The listing builds one solid part. Answer for the finished solid, in the listing's coordinates (mm). Face numbers are marked on the shaded views. Round coordinates to 2 decimals unless told otherwise and drop trailing zeros. Order: outer loops, then holes, each group sorted by start corner. A loop starts at its lowest first (then second) coordinate and runs counter-clockwise, first axis right, second up. Notation, with made-up numbers: (67.5, 25) - (73.5, 25) arc R22 ccw to (73.5, 33) - close; hole circle Ø10 at (-13.5, 40.25). An arc over 180 degrees is marked (long way). One line per item, written item: value. Start each with the question number.
1. Section B-B, the plane x = -24 is taken. Give the vertices of the cut face in (y, z).
2. Section A-A, the plane z = 24.5 is taken. Give the vertices of the cut face in (x, y).
3. Straight lines are drawn through the part: line 1 (Z direction, x = 27, y = -2.75); line 2 (Z direction, x = -12.5, y = -18.25); line 3 (Z direction, x = -11, y = -7.5). For each, find the intervals that lie inside material, in ascending order.
4. Section C-C, the plane y = -19.25 is taken. Count the separate pieces of the cut face and the enclosed holes in it, then the cut area to 3 significant figures.
5. For a pull along Z with two mould halves and no side action, classify the marked faces 1, 2, 3 and 4 as released by +Z, released by -Z, zero draft, split by the parting line, or undercut.
6. Section D-D, the plane x = 42.5 is taken. Give the vertices of the cut face in (y, z).
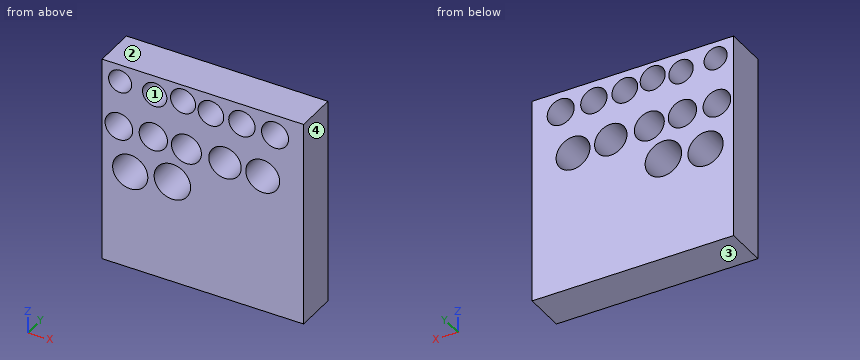
from build123d import *

# Parameters (mm, degrees)
F0_W     = 123.113498
F0_H     = 126.693976
F1_DEPTH = 25.4
F3_D     = 14.1
F4_D     = 14.9
F5_D     = 15.3
F6_D     = 15.7
F7_D     = 16.1
F8_D     = 16.5
F9_D     = 16.9
F10_D    = 17.3
F11_D    = 18.3
F12_D    = 19.8
F13_D    = 20.7
F14_D    = 21.5
F15_D    = 22.3


with BuildPart() as f1:
    # F0 (on Front) → F1 (new body)
    with BuildSketch(Plane.XZ):
        with Locations((2.891928, -3.167348)):
            Rectangle(F0_W, F0_H)
    extrude(amount=F1_DEPTH)

    # F3 (through all)
    with Locations(Plane.XZ.offset(25.4)):
        with Locations((-47.647953, 49.713619)):
            Hole(F3_D / 2)

    # F4 (through all)
    with Locations(Plane.XZ.offset(25.4)):
        with Locations((-26.540603, 48.396926)):
            Hole(F4_D / 2)

    # F5 (through all)
    with Locations(Plane.XZ.offset(25.4)):
        with Locations((-9.222592, 50.100338)):
            Hole(F5_D / 2)

    # F6 (through all)
    with Locations(Plane.XZ.offset(25.4)):
        with Locations((7.811517, 48.113026)):
            Hole(F6_D / 2)

    # F7 (through all)
    with Locations(Plane.XZ.offset(25.4)):
        with Locations((26.720595, 47.939809)):
            Hole(F7_D / 2)

    # F8 (through all)
    with Locations(Plane.XZ.offset(25.4)):
        with Locations((46.989974, 47.545221)):
            Hole(F8_D / 2)

    # F9 (through all)
    with Locations(Plane.XZ.offset(25.4)):
        with Locations((-48.436428, 20.943279)):
            Hole(F9_D / 2)

    # F10 (through all)
    with Locations(Plane.XZ.offset(25.4)):
        with Locations((-27.392309, 21.426253)):
            Hole(F10_D / 2)

    # F11 (through all)
    with Locations(Plane.XZ.offset(25.4)):
        with Locations((-7.154659, 20.386403)):
            Hole(F11_D / 2)

    # F12 (through all)
    with Locations(Plane.XZ.offset(25.4)):
        with Locations((16.401133, 19.650284)):
            Hole(F12_D / 2)

    # F13 (through all)
    with Locations(Plane.XZ.offset(25.4)):
        with Locations((39.46618, 18.914167)):
            Hole(F13_D / 2)

    # F14 (through all)
    with Locations(Plane.XZ.offset(25.4)):
        with Locations((-41.506853, -5.623117)):
            Hole(F14_D / 2)

    # F15 (through all)
    with Locations(Plane.XZ.offset(25.4)):
        with Locations((-15.742708, -3.169389)):
            Hole(F15_D / 2)


solid = f1.part
Answer list:
1. outline: (-25.4, -66.51) - (0, -66.51) - (0, -10.66) - (-25.4, -10.66) - close; (-25.4, 4.32) - (0, 4.32) - (0, 13.47) - (-25.4, 13.47) - close; (-25.4, 29.38) - (0, 29.38) - (0, 41.39) - (-25.4, 41.39) - close; (-25.4, 55.4) - (0, 55.4) - (0, 60.18) - (-25.4, 60.18) - close
2. outline: (-58.66, -25.4) - (-56.1, -25.4) - (-56.1, 0) - (-58.66, 0) - close; (-40.77, -25.4) - (-35.48, -25.4) - (-35.48, 0) - (-40.77, 0) - close; (-19.31, -25.4) - (-15.33, -25.4) - (-15.33, 0) - (-19.31, 0) - close; (1.02, -25.4) - (7.77, -25.4) - (7.77, 0) - (1.02, 0) - close; (25.03, -25.4) - (30.75, -25.4) - (30.75, 0) - (25.03, 0) - close; (48.18, -25.4) - (64.45, -25.4) - (64.45, 0) - (48.18, 0) - close
3. line 1: z = -66.51 to 39.89, 55.98 to 60.18
3. line 2: z = -66.51 to -13.84, 7.5 to 12.96, 27.81 to 43.19, 57.01 to 60.18
3. line 3: z = -66.51 to -13.26, 6.92 to 12.08, 28.69 to 42.66, 57.54 to 60.18
4. separate pieces: 1
4. enclosed holes: 13
4. area: 12,400 mm²
5. face 1: undercut
5. face 2: released by +Z
5. face 3: released by -Z
5. face 4: zero draft
6. outline: (-25.4, -66.51) - (0, -66.51) - (0, 9.02) - (-25.4, 9.02) - close; (-25.4, 28.81) - (0, 28.81) - (0, 40.62) - (-25.4, 40.62) - close; (-25.4, 54.47) - (0, 54.47) - (0, 60.18) - (-25.4, 60.18) - close
